Can you work these out from the model? Positions are in its coordinate system, mm. Face numbers are marked on the shaded views. Round coordinates to 2 decimals unless told otherwise and drop trailing zeros. Write each loop counter-clockwise with the first axis right and the second up, starting at its lowest first coordinate (ties: lowest second). Pieces come first, ordered by that corner, then holes.
Q1. I'm going to push flat-ended pins straight in: pin 1 Ø2 at (y, z) = (-19.5, 2.5) entering from +X; pin 2 Ø3 at (x, y) = (2, -25.5) entering from +Z; pin 3 Ø4 at (y, z) = (-18.5, 6) entering from -X; pin 4 Ø8 at (x, z) = (8, 7) entering from +Y. Where does each tip first touch, or does it pass through?
Q2. If we section it at B-B (x = 0): Please give me the cut outline in (y, z).
Q3. Please list where these lines run through material, in increasing order: line 1 along Z through (x, y) = (0, -7); line 2 along X through (y, z) = (-25.5, -5.75); line 3 along Z through (x, y) = (-4.25, -8.5).
Q4. If we section it at A-A (z = 0): Please give me the cut outline in (x, y), plus the area to 3 significant figures.
Q5. We'd pull the mould along X, two halves only. Please class the marked faces 1, 2 and 3: +X half, -X half, draft (parallel to the pull), parting line (faces both ways), or undercut.
Q6. If we section it at C-C (y = -13.5): Please give me the cut outline in (x, z), plus the area to 3 significant figures.
from build123d import *

# Parameters (mm, degrees)
F0_R     = 15
F0_R_2   = 12.5
F1_DEPTH = 3
F0_R_3   = 10
F2_DEPTH = 31
F3_SIZE  = 0.25


with BuildPart() as f1:
    # F0 (on Front) → F1 (new body)
    with BuildSketch(Plane.XZ):
        Circle(F0_R)
        Circle(F0_R_2, mode=Mode.SUBTRACT)
    extrude(amount=F1_DEPTH)

    # F0 (on Front) → F2 (join)
    with BuildSketch(Plane.XZ):
        Circle(F0_R_2)
        Circle(F0_R_3, mode=Mode.SUBTRACT)
    extrude(amount=F2_DEPTH)

    # F3
    f3_edges = [f1.edges().sort_by_distance(p)[0] for p in [
        (-12.5, -31, 0),
        (-10, -31, 0),
        (-15, 0, 0),
        (-10, 0, 0),
        (-15, -3, 0),
    ]]
    chamfer(f3_edges, length=F3_SIZE)


solid = f1.part
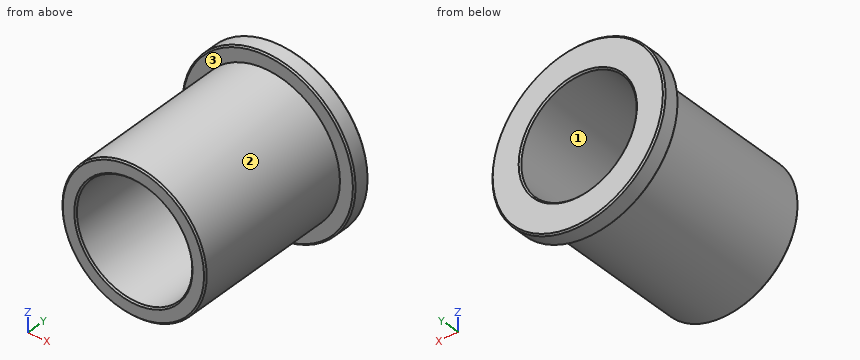
A:
1. pin 1: stops at x = 12.41
1. pin 2: stops at z = 12.49
1. pin 3: stops at x = -11.84
1. pin 4: stops at y = 0
2. outline: (-31, -12.25) - (-30.75, -12.5) - (-3, -12.5) - (-3, -14.75) - (-2.75, -15) - (-0.25, -15) - (0, -14.75) - (0, -10.25) - (-0.25, -10) - (-30.75, -10) - (-31, -10.25) - close; (-31, 10.25) - (-30.75, 10) - (-0.25, 10) - (0, 10.25) - (0, 14.75) - (-0.25, 15) - (-2.75, 15) - (-3, 14.75) - (-3, 12.5) - (-30.75, 12.5) - (-31, 12.25) - close
3. line 1: z = -12.5 to -10, 10 to 12.5
3. line 2: x = -11.1 to -8.18, 8.18 to 11.1
3. line 3: z = -11.76 to -9.05, 9.05 to 11.76
4. outline: (-15, -2.75) - (-14.75, -3) - (-12.5, -3) - (-12.5, -30.75) - (-12.25, -31) - (-10.25, -31) - (-10, -30.75) - (-10, -0.25) - (-10.25, 0) - (-14.75, 0) - (-15, -0.25) - close; (10, -30.75) - (10.25, -31) - (12.25, -31) - (12.5, -30.75) - (12.5, -3) - (14.75, -3) - (15, -2.75) - (15, -0.25) - (14.75, 0) - (10.25, 0) - (10, -0.25) - close
4. area: 170 mm2
5. face 1: undercut
5. face 2: parting line
5. face 3: draft
6. outline: circle Ø25 at (0, 0); hole circle Ø20 at (0, 0)
6. area: 177 mm2
